from build123d import *

# Parameters (mm, degrees)
F0_W     = 127
F0_H     = 127
F1_DEPTH = 254
F3_D     = 38.1
F4_R     = 25.4
F5_SIZE  = 25.4


with BuildPart() as f1:
    # F0 (on Front) → F1 (new body)
    with BuildSketch(Plane.XZ):
        with Locations((63.5, -63.5)):
            Rectangle(F0_W, F0_H)
    extrude(amount=F1_DEPTH)

    # F3 (through all)
    with Locations(Plane(origin=(0, 0, 0), x_dir=(1, 0, 0), z_dir=(0, 1, 0))):
        with Locations((63.5, 63.5)):
            Hole(F3_D / 2)

    # F4
    f4_edges = [f1.edges().sort_by_distance(p)[0] for p in [
        (127, -127, 0),
        (0, -127, 0),
    ]]
    fillet(f4_edges, radius=F4_R)

    # F5
    f5_edges = [f1.edges().sort_by_distance(p)[0] for p in [
        (127, -127, -127),
        (0, -127, -127),
    ]]
    chamfer(f5_edges, length=F5_SIZE)


solid = f1.part
The model under review builds one solid part; all positions refer to its coordinate system, in mm. Give positions to 0.01 mm unless a question says otherwise; leave off trailing zeros. Order: outer loops, then holes, each group sorted by start corner. A loop starts at its lowest first (then second) coordinate and runs counter-clockwise, first axis right, second up. Notation, with made-up numbers: (-10, -25.75) -> (21, -25.75) arc R18 cw to (21, -2.75) -> close; hole circle Ø9 at (77, 37). An arc over 180 degrees is marked (long way). Write item = value, one per line. Start each with the question number.
(1) Take a section at B-B (z = -70.5). Write out the cut boundary in (x, y), plus the area to 3 significant figures.
(2) For L1, parallel to X at y = -51, z = -63; L2, parallel to Z at x = 63.5, y = -97; L3, parallel to Z at x = 71, y = -98, list the stretches that pass through material, from the lowest coordinate up. Write a range as from..to.
(3) Take a section at D-D (z = -119). Write out the cut boundary in (x, y).
(4) Take a section at C-C (y = -170.5). Write out the cut boundary in (x, z).
(5) Take a section at A-A (x = 63.5). Write out the cut boundary in (y, z), plus the area to 3 significant figures.
(6) Draft analysis for pull direction Z (two halves, no side actions). For faces 1 (the flat face through (48, 0, -48)), 2 (the cylindrical face through (78.62, -128.78, -51.91)), 3 (the cylindrical face through (7.24, -128.78, -7.64)), state which applies: +Z half, -Z half, draft (parallel to the pull), parting line (faces both ways), or undercut.
Returned:
q1.outline = (0, -254) -> (45.78, -254) -> (45.78, 0) -> (0, 0) -> close; (81.22, -254) -> (127, -254) -> (127, 0) -> (81.22, 0) -> close
q1.area = 23,300 mm²
q2.L1 = 0..44.46, 82.54..127
q2.L2 = -127..-82.55, -44.45..0
q2.L3 = -127..-81.01, -45.99..0
q3.outline = (17.4, -254) -> (109.6, -254) -> (109.6, 0) -> (17.4, 0) -> close
q4.outline = (0, -101.6) -> (25.4, -127) -> (101.6, -127) -> (127, -101.6) -> (127, -25.4) arc R25.4 ccw to (101.6, 0) -> (25.4, 0) arc R25.4 ccw to (0, -25.4) -> close; hole circle Ø38.1 at (63.5, -63.5)
q5.outline = (-254, -127) -> (0, -127) -> (0, -82.55) -> (-254, -82.55) -> close; (-254, -44.45) -> (0, -44.45) -> (0, 0) -> (-254, 0) -> close
q5.area = 22,600 mm²
q6.face_1 = draft
q6.face_2 = undercut
q6.face_3 = +Z half
